Verification items for this drawing (mm, ordinates from the low corner). Round coordinates to 2 decimals unless told otherwise and drop trailing zeros. Loops run counter-clockwise (first coordinate to the right, second up) from the corner with the lowest first, then second, coordinate; pieces in that order, holes last. Notation, with made-up numbers: (64.5, 18) - (87.5, 18) arc R6 ccw to (87.5, 26) - close; hole circle Ø6 at (72, -29.75). An arc over 180 degrees is marked (long way). Answer in a Markdown table with one row per item. Add a question column.
(1) Gauge pin test, flat ends, axial feed: pin 1 (1.2 mm diameter, centred on x = 8.5, z = 1.5, fed in from +Y); pin 2 (2 mm diameter, centred on x = 91, z = 2, fed in from +Y); pin 3 (1.5 mm diameter, centred on y = 30.5, z = 3.5, fed in from -X). Record the tip position at first contact, or that the pin passes through.
(2) Cross-section at A-A on x = 82. Enter the section's corners in (y, z).
(3) Cross-section at B-B on y = 52. Enter the section's corners in (x, z).
(4) Thickness scan on line 1 along Y through (x, z) = (65, 0.2); line 2 along X through (y, z) = (30, 3.3). Record the ranges inside material, lowest first.
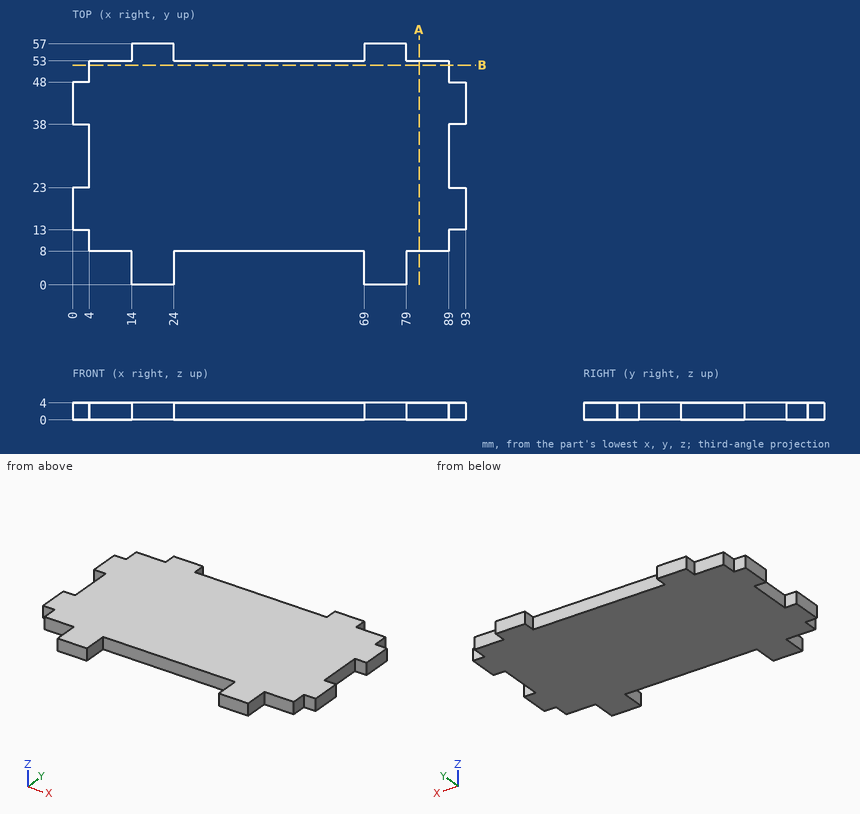
Answers:
| question | item | result |
|---|---|---|
| 1 | pin 1 | stops at y = 53 |
| 1 | pin 2 | stops at y = 48 |
| 1 | pin 3 | stops at x = 4 |
| 2 | outline | (8, 0) - (53, 0) - (53, 4) - (8, 4) - close |
| 3 | outline | (4, 0) - (89, 0) - (89, 4) - (4, 4) - close |
| 4 | line 1 | y = 8 to 53 |
| 4 | line 2 | x = 4 to 89 |
